from build123d import *

# Parameters (mm, degrees)
CROQUIS1_R                               = 12.2
SALIENTE_EXTRUIR1_DEPTH                  = 31
CROQUIS2_R                               = 13.5
SALIENTE_EXTRUIR2_DEPTH                  = 27
CROQUIS3_R                               = 2.15
CROQUIS3_R_2                             = 1
SALIENTE_EXTRUIR3_DEPTH                  = 6.5
CHAFL_N2_SIZE                            = 0.5
REDONDEO1_R                              = 0.5
CROQUIS5_R                               = 2.15
CROQUIS5_R_2                             = 1
SALIENTE_EXTRUIR4_DEPTH                  = 7
SALIENTE_EXTRUIR4_DIRECTION_2_REACH      = 73.214
SALIENTE_EXTRUIR4_DIRECTION_2_END_RADIUS = 13.5
CHAFL_N3_SIZE                            = 0.3
CROQUIS6_R                               = 3
SALIENTE_EXTRUIR5_DEPTH                  = 2
REDONDEO2_R                              = 1


with BuildPart() as part:
    # Croquis1 → Saliente-Extruir1 (new body)
    with BuildSketch(Plane.XY):
        Circle(CROQUIS1_R)
    extrude(amount=SALIENTE_EXTRUIR1_DEPTH)

    # Croquis2 → Saliente-Extruir2 (add)
    with BuildSketch(Plane.XY.offset(31)):
        Circle(CROQUIS2_R)
    extrude(amount=SALIENTE_EXTRUIR2_DEPTH)

    # Croquis3 → Saliente-Extruir3 (add)
    with BuildSketch(Plane.XY.offset(58)):
        with Locations(Location((0, 0, 0), (0, 0, 180))):
            Circle(CROQUIS3_R)
        with Locations(Location((0, 0, 0), (0, 0, 180))):
            Circle(CROQUIS3_R_2, mode=Mode.SUBTRACT)
    extrude(amount=SALIENTE_EXTRUIR3_DEPTH)

    # Chaflán2
    chafl_n2_edges = [part.edges().sort_by_distance(p)[0] for p in [
        (2.15, 0, 64.5),
    ]]
    chamfer(chafl_n2_edges, length=CHAFL_N2_SIZE)

    # Redondeo1
    redondeo1_edges = [part.edges().sort_by_distance(p)[0] for p in [
        (2.15, 0, 58),
    ]]
    fillet(redondeo1_edges, radius=REDONDEO1_R)

    # Croquis5 → Saliente-Extruir4 (add)
    with BuildSketch(Plane(origin=(0, 13.5, 0), x_dir=(1, 0, 0), z_dir=(0, 1, 0))):
        with Locations(Location((0, -35.85, 0), (0, 0, 90))):
            Circle(CROQUIS5_R)
        with Locations(Location((0, -35.85, 0), (0, 0, 270))):
            Circle(CROQUIS5_R_2, mode=Mode.SUBTRACT)
    extrude(amount=SALIENTE_EXTRUIR4_DEPTH)

    # Saliente-Extruir4 direction 2: up to this cylinder (the profile starts outside it)
    saliente_extruir4_direction_2_end = Plane(origin=(0, 0, 37.939189), z_dir=(0, 0, -1)) * Cylinder(SALIENTE_EXTRUIR4_DIRECTION_2_END_RADIUS, 174.428, mode=Mode.PRIVATE)
    # Croquis5 → Saliente-Extruir4 direction 2 (add, up to the surface)
    with BuildSketch(Plane(origin=(0, 13.5, 0), x_dir=(1, 0, 0), z_dir=(0, 1, 0)), mode=Mode.PRIVATE) as saliente_extruir4_direction_2_sk1:
        with Locations(Location((0, -35.85, 0), (0, 0, 90))):
            Circle(CROQUIS5_R)
        with Locations(Location((0, -35.85, 0), (0, 0, 270))):
            Circle(CROQUIS5_R_2, mode=Mode.SUBTRACT)
    saliente_extruir4_direction_2_tool1 = extrude(saliente_extruir4_direction_2_sk1.sketch, amount=-SALIENTE_EXTRUIR4_DIRECTION_2_REACH, mode=Mode.PRIVATE) - saliente_extruir4_direction_2_end
    add(saliente_extruir4_direction_2_tool1.solids().sort_by_distance((0, 13.5, 37.939189))[0])
    add(saliente_extruir4_direction_2_tool1.solids().sort_by_distance((0, 13.5, 37.939189))[1])

    # Chaflán3
    chafl_n3_edges = [part.edges().sort_by_distance(p)[0] for p in [
        (0, 20.5, 38),
    ]]
    chamfer(chafl_n3_edges, length=CHAFL_N3_SIZE)

    # Croquis6 → Saliente-Extruir5 (add)
    with BuildSketch(Plane(origin=(0, 0, 0), x_dir=(-1, 0, 0), z_dir=(0, 0, -1))):
        Circle(CROQUIS6_R)
    extrude(amount=SALIENTE_EXTRUIR5_DEPTH)

    # Redondeo2
    redondeo2_edges = [part.edges().sort_by_distance(p)[0] for p in [
        (3, 0, -2),
    ]]
    fillet(redondeo2_edges, radius=REDONDEO2_R)


solid = part.part
Can you work these out from the model? Positions are in its coordinate system, mm. A direction names the side the tool comes from. Coordinates: 2 decimals unless noted, no trailing zeros. Order: outer loops, then holes, each group sorted by start corner. A loop starts at its lowest first (then second) coordinate and runs counter-clockwise, first axis right, second up. Notation, with made-up numbers: (3.5, 27.25) - (12.5, 27.25) arc R24 cw to (12.5, 42.25) - close; hole circle Ø6 at (-28.5, 66). An arc over 180 degrees is marked (long way). Answer as a JSON object with one key per item and string values. Group by question number.
Q1. On a 3-axis mill with a long thin cutter (end or side, diameter ignored), from which of +Z, -Z, +X, -X, +Y, -Y can I reach the whole of each face in a straight line? I mean faces 1 (the face through (2.15, -0.09, 61.21)), 2 (the face through (-0.65, 16.72, 33.8)), 3 (the face through (-3, -12, 31)). Say none if no direction works.
Q2. I need wall thicknesses on line 1 (X direction, y = 19, z = 35.85); line 2 (X direction, y = 17, z = 35). Which ranges of each line are inside material? Lowest first, please. Write a range as from..to.
Q3. Will these pins go through, and if not, where does the flat tip stop? P1, Ø8, axis at x = 6, y = 5.5, coming from the +Z side; P2, Ø3, axis at y = 1.5, z = 26.5, coming from the -X side; P3, Ø12, axis at x = 10.5, z = 46, coming from the +Y side.
Q4. Imagine slicing it at C-C (y = 18). Please give me the cut outline in (x, z), and give its area (3 significant figures).
Q5. Imagine slicing it at D-D (x = 4.25). Please give me the cut outline in (y, z).
Q6. Imagine slicing it at A-A (y = 0). Please give me the cut outline in (x, z), and give its area (3 significant figures).
Q7. Imagine slicing it at B-B (z = 35.85). Please give me the cut outline in (x, y).
Q8. We'd pull the mould along Z, two halves only. Please class faces 4 (the face through (-12.19, 0.54, 15.28)), 5 (the face through (0, 0, 58)), 6 (the face through (0.04, 16.93, 34.85)): +Z half, -Z half, draft (parallel to the pull), parting line (faces both ways), or undercut.
Determined:
{
 "1": {"face 1": "+Z", "face 2": "+Y", "face 3": "-Z"},
 "2": {"line 1": "x = -2.15..-1, 1..2.15", "line 2": "x = -1.97..-0.53, 0.53..1.97"},
 "3": {"P1": "stops at z = 58", "P2": "stops at x = -12.2", "P3": "stops at y = 12.73"},
 "4": {"outline": "circle Ø4.3 at (0, 35.85); hole circle Ø2 at (0, 35.85)", "area": "11.4 mm2"},
 "5": {"outline": "(-12.81, 31) - (-11.44, 31) - (-11.44, 0) - (11.44, 0) - (11.44, 31) - (12.81, 31) - (12.81, 58) - (-12.81, 58) - close"},
 "6": {"outline": "(-13.5, 31) - (-12.2, 31) - (-12.2, 0) - (-3, 0) - (-3, -1) arc R1 ccw to (-2, -2) - (2, -2) arc R1 ccw to (3, -1) - (3, 0) - (12.2, 0) - (12.2, 31) - (13.5, 31) - (13.5, 58) - (2.65, 58) arc R0.5 cw to (2.15, 58.5) - (2.15, 64) - (1.65, 64.5) - (1, 64.5) - (1, 58) - (-1, 58) - (-1, 64.5) - (-1.65, 64.5) - (-2.15, 64) - (-2.15, 58.5) arc R0.5 cw to (-2.65, 58) - (-13.5, 58) - close", "area": "1,510 mm2"},
 "7": {"outline": "(-2.15, 13.33) arc R13.5 ccw (long way) to (2.15, 13.33) - (2.15, 20.2) - (1.85, 20.5) - (1, 20.5) - (1, 13.46) arc R13.5 ccw to (-1, 13.46) - (-1, 20.5) - (-1.85, 20.5) - (-2.15, 20.2) - close"},
 "8": {"face 4": "draft", "face 5": "+Z half", "face 6": "undercut"}
}
